```python
from build123d import *

# Parameters (mm, degrees)
F_1P5MM_64_START              = -32
F_1P5MM_64_DEPTH              = 64
CUT_EXTRUDE_M3_1_DEPTH        = 100
CUT_EXTRUDE_M3_1_DEPTH_BACK   = 100
SKETCH_2_R                    = 1.65
CUT_EXTRUDE_M3_1_2_DEPTH      = 100
CUT_EXTRUDE_M3_1_2_DEPTH_BACK = 100
SKETCH_4_R                    = 1.65
CUT_EXTRUDE_M3_1_3_DEPTH      = 100
CUT_EXTRUDE_M3_1_3_DEPTH_BACK = 100
SKETCH_5_R                    = 1.65
CUT_EXTRUDE_M3_1_4_DEPTH      = 100
CUT_EXTRUDE_M3_1_4_DEPTH_BACK = 100
SKETCH_7_R                    = 1.65
FDM_R2_R                      = 2
FDM_3MM_16_START              = -17.5
FDM_3MM_16_DEPTH              = 3
FDM_3MM_0_START               = -1.5
FDM_3MM_0_DEPTH               = 3
FDM_3MM_16_START_2            = 14.5
FDM_3MM_16_2_DEPTH            = 3


with BuildPart() as part:
    # 草图1 → 1p5mm铝合金直角座_宽64 (new body)
    with BuildSketch(Plane.XY.offset(F_1P5MM_64_START)):
        Polygon((0, 0), (16, 0), (16, 4), (4, 4), (4, 14), (0, 14), align=None)
    extrude(amount=F_1P5MM_64_DEPTH)

    # 草图2 → Cut-Extrude M3_-1 (cut, two sides: drawn at the far end of the back side and taken through both)
    with BuildSketch(Plane(origin=(0, 0, 0), x_dir=(0, 0, -1), z_dir=(1, 0, 0)).offset(-CUT_EXTRUDE_M3_1_DEPTH_BACK)):
        with Locations((24, 10)):
            Circle(SKETCH_2_R)
    extrude(amount=CUT_EXTRUDE_M3_1_DEPTH + CUT_EXTRUDE_M3_1_DEPTH_BACK, mode=Mode.SUBTRACT)

    # 草图4 → Cut-Extrude M3_-1 2 (cut, two sides: drawn at the far end of the back side and taken through both)
    with BuildSketch(Plane(origin=(0, 0, 0), x_dir=(1, 0, 0), z_dir=(0, 1, 0)).offset(-CUT_EXTRUDE_M3_1_2_DEPTH_BACK)):
        with Locations(Location((12, 28, 0), (0, 0, 270))):
            Circle(SKETCH_4_R)
    extrude(amount=CUT_EXTRUDE_M3_1_2_DEPTH + CUT_EXTRUDE_M3_1_2_DEPTH_BACK, mode=Mode.SUBTRACT)

    # 草图5 → Cut-Extrude M3_1 3 (cut, two sides: drawn at the far end of the back side and taken through both)
    with BuildSketch(Plane(origin=(0, 0, 0), x_dir=(0, 0, -1), z_dir=(1, 0, 0)).offset(-CUT_EXTRUDE_M3_1_3_DEPTH_BACK)):
        with Locations((-24, 10)):
            Circle(SKETCH_5_R)
    extrude(amount=CUT_EXTRUDE_M3_1_3_DEPTH + CUT_EXTRUDE_M3_1_3_DEPTH_BACK, mode=Mode.SUBTRACT)

    # 草图7 → Cut-Extrude M3_1 4 (cut, two sides: drawn at the far end of the back side and taken through both)
    with BuildSketch(Plane(origin=(0, 0, 0), x_dir=(1, 0, 0), z_dir=(0, 1, 0)).offset(-CUT_EXTRUDE_M3_1_4_DEPTH_BACK)):
        with Locations(Location((12, -28, 0), (0, 0, 270))):
            Circle(SKETCH_7_R)
    extrude(amount=CUT_EXTRUDE_M3_1_4_DEPTH + CUT_EXTRUDE_M3_1_4_DEPTH_BACK, mode=Mode.SUBTRACT)

    # FDM根部内圆角_R2
    fdm_r2_edges = [part.edges().sort_by_distance(p)[0] for p in [
        (4, 4, 0),
    ]]
    fillet(fdm_r2_edges, radius=FDM_R2_R)

    # 草图8 → FDM__3mm_-16 (add)
    with BuildSketch(Plane.XY.offset(FDM_3MM_16_START)):
        Polygon((3.5, 3.5), (14, 3.5), (3.5, 12.5), align=None)
    extrude(amount=FDM_3MM_16_DEPTH)

    # 草图9 → FDM三角加强筋_3mm_0 (add)
    with BuildSketch(Plane.XY.offset(FDM_3MM_0_START)):
        Polygon((3.5, 3.5), (14, 3.5), (3.5, 12.5), align=None)
    extrude(amount=FDM_3MM_0_DEPTH)

    # 草图10 → FDM__3mm_16 2 (add)
    with BuildSketch(Plane.XY.offset(FDM_3MM_16_START_2)):
        Polygon((3.5, 3.5), (14, 3.5), (3.5, 12.5), align=None)
    extrude(amount=FDM_3MM_16_2_DEPTH)


solid = part.part
```
Geometry check sheet. Reference: the model listing, model coordinates, mm. A direction names the side the tool comes from. Round coordinates to 2 decimals unless told otherwise and drop trailing zeros. Loops run counter-clockwise (first coordinate to the right, second up) from the corner with the lowest first, then second, coordinate; pieces in that order, holes last. Notation, with made-up numbers: M -34.75,35 L 16.25,35 A22 cw 16.25,53 Z; hole C 26.25,66 d6. An arc over 180 degrees is marked long. Return JSON: item names as keys, results as strings. Group by question number.
(1) Section check A-A, the plane z = -24. Enter the section's corners in (x, y).
(2) Set-up check for faces 4 (the face through (4.6, 4.57, -24.65)), 5 (the face through (4.6, 4.57, 8.09)), 6 (the face through (2, 14, 0)): record each of +Z, -Z, +X, -X, +Y, -Y from which the full face is reachable in a straight line by a thin tool's end or side.
(3) Scan lines: line 1 along Z through (x, y) = (1.45, 10); line 2 along Z through (x, y) = (12, 2.5); line 3 along Y through (x, z) = (3.05, -24). Record each from-to range of solid material in increasing order. Write a range as [from, to].
(4) Section check D-D, the plane x = 15.25. Enter the section's corners in (y, z).
(5) Section check C-C, the plane z = 0. Enter the section's corners in (x, y).
(6) Go/stop test with flat-tipped pins: pin 1 (6.5 mm diameter, centred on x = 8, y = 7.5, fed in from -Z); pin 2 (5 mm diameter, centred on x = 9.5, z = 9, fed in from +Y); pin 3 (1.5 mm diameter, centred on y = 7, z = -6, fed in from +X). Record where each tip stops, or that it passes through.
(7) Section check B-B, the plane y = 10. Enter the section's corners in (x, z).
(8) Mould release check, pull along Y, two halves, no side actions. Record for faces 1 (the face through (8.774, 7.979, -16.021)), 2 (the face through (1.97, 10.07, -22.35)), 3 (the face through (7, 6, -14.5)): pulls with the +Y half, pulls with the -Y half, needs draft (parallel to the pull), parting line crosses it, or undercut.
Data:
{
 "1": {"outline": "M 0,0 L 16,0 L 16,4 L 6,4 A2 cw 4,6 L 4,8.35 L 0,8.35 Z; M 0,11.65 L 4,11.65 L 4,14 L 0,14 Z"},
 "2": {"face 4": "-Z, +X, +Y", "face 5": "+X, +Y", "face 6": "+Z, -Z, +X, -X, +Y"},
 "3": {"line 1": "[-32, -25.65], [-22.35, 22.35], [25.65, 32]", "line 2": "[-32, -29.65], [-26.35, 26.35], [29.65, 32]", "line 3": "[0, 8.35], [11.65, 14]"},
 "4": {"outline": "M 0,-32 L 4,-32 L 4,32 L 0,32 Z"},
 "5": {"outline": "M 0,0 L 16,0 L 16,4 L 13.42,4 L 4,12.07 L 4,14 L 0,14 Z"},
 "6": {"pin 1": "z = -17.5", "pin 2": "y = 4", "pin 3": "x = 4"},
 "7": {"outline": "M 0,-32 L 4,-32 L 4,-25.65 L 0,-25.65 Z; M 0,-22.35 L 4,-22.35 L 4,-17.5 L 6.42,-17.5 L 6.42,-14.5 L 4,-14.5 L 4,-1.5 L 6.42,-1.5 L 6.42,1.5 L 4,1.5 L 4,14.5 L 6.42,14.5 L 6.42,17.5 L 4,17.5 L 4,22.35 L 0,22.35 Z; M 0,25.65 L 4,25.65 L 4,32 L 0,32 Z"},
 "8": {"face 1": "pulls with the +Y half", "face 2": "undercut", "face 3": "needs draft"}
}
